Can you work these out from the model? Positions are in its coordinate system, mm. A direction names the side the tool comes from. Round coordinates to 2 decimals unless told otherwise and drop trailing zeros. Order: outer loops, then holes, each group sorted by start corner. A loop starts at its lowest first (then second) coordinate and runs counter-clockwise, first axis right, second up.
from build123d import *

# Parameters (mm, degrees)
SKETCH1_W           = 31.5
SKETCH1_H           = 30.3
SKETCH1_W_2         = 25.5
SKETCH1_H_2         = 24.3
BOSS_EXTRUDE1_DEPTH = 6
SKETCH2_W           = 31.5
SKETCH2_H           = 30.3
BOSS_EXTRUDE2_DEPTH = 2
CUT_EXTRUDE1_DEPTH  = 61
BOSS_EXTRUDE3_DEPTH = 2
SKETCH5_W           = 4
SKETCH5_H           = 27.3
BOSS_EXTRUDE4_DEPTH = 38
CUT_EXTRUDE2_DEPTH  = 38
SKETCH7_R           = 2.6
CUT_EXTRUDE3_DEPTH  = 38
CUT_EXTRUDE4_DEPTH  = 38
FILLET1_R           = 10


with BuildPart() as part:
    # Sketch1 → Boss-Extrude1 (new body)
    with BuildSketch(Plane.XY):
        with Locations((12.75, 12.15)):
            Rectangle(SKETCH1_W, SKETCH1_H)
        with Locations((12.75, 12.15)):
            Rectangle(SKETCH1_W_2, SKETCH1_H_2, mode=Mode.SUBTRACT)
    extrude(amount=BOSS_EXTRUDE1_DEPTH)

    # Sketch2 → Boss-Extrude2 (add)
    with BuildSketch(Plane(origin=(0, 0, 0), x_dir=(-1, 0, 0), z_dir=(0, 0, -1))):
        with Locations((-12.75, 12.15)):
            Rectangle(SKETCH2_W, SKETCH2_H)
    extrude(amount=BOSS_EXTRUDE2_DEPTH)

    # Sketch3 → Cut-Extrude1 (cut)
    with BuildSketch(Plane.XY.offset(6)):
        Polygon((-3, 24.391972576), (-3, 27.3), (28.5, 27.3), (28.5, 24.391972576), (28.5, 24.3), (0, 24.3), (-3, 24.3), align=None)
    extrude(amount=-CUT_EXTRUDE1_DEPTH, mode=Mode.SUBTRACT)

    # Sketch4 → Boss-Extrude3 (add)
    with BuildSketch(Plane.XY.offset(6)):
        with BuildLine():
            Line((-3, 24.3), (5.5, 24.3))
            Line((5.5, 24.3), (5.5, 8.75))
            ThreePointArc((5.5, 8.75), (12.75, 1.5), (20, 8.75))
            Line((20, 8.75), (20, 24.3))
            Line((20, 24.3), (28.5, 24.3))
            Line((28.5, 24.3), (28.5, -3))
            Line((28.5, -3), (-3, -3))
            Line((-3, -3), (-3, 24.3))
        make_face()
    extrude(amount=BOSS_EXTRUDE3_DEPTH)

    # Sketch5 → Boss-Extrude4 (add)
    with BuildSketch(Plane(origin=(0, 0, -2), x_dir=(-1, 0, 0), z_dir=(0, 0, -1))):
        with Locations((-26.5, 10.65)):
            Rectangle(SKETCH5_W, SKETCH5_H)
    extrude(amount=BOSS_EXTRUDE4_DEPTH)

    # Sketch6 → Cut-Extrude2 (cut)
    with BuildSketch(Plane.ZY.offset(-24.5)):
        with BuildLine():
            Line((-2, -3), (-40, -3))
            Line((-40, -3), (-40, 24.3))
            Line((-40, 24.3), (-2, 24.3))
            Line((-2, 24.3), (-17.826401454, 15.23386068))
            ThreePointArc((-17.826401454, 15.23386068), (-18.562622883, 14.501365189), (-18.832265792, 13.498437306))
            Line((-18.832265792, 13.498437306), (-18.832265792, 7.801562694))
            ThreePointArc((-18.832265792, 7.801562694), (-18.562622883, 6.798634811), (-17.826401454, 6.06613932))
            Line((-17.826401454, 6.06613932), (-2, -3))
        make_face()
    extrude(amount=-CUT_EXTRUDE2_DEPTH, mode=Mode.SUBTRACT)

    # Sketch7 → Cut-Extrude3 (cut)
    with BuildSketch(Plane.ZY.offset(-24.5)):
        with Locations(Location((-10.416132896, 10.65, 0), (0, 0, 270))):
            Circle(SKETCH7_R)
    extrude(amount=-CUT_EXTRUDE3_DEPTH, mode=Mode.SUBTRACT)

    # Sketch8 → Cut-Extrude4 (cut)
    with BuildSketch(Plane.ZY.offset(-24.5)):
        with BuildLine():
            ThreePointArc((-11.252656387, 0.614520451), (-15.36913817, 13.404749459), (-6.531723112, 23.52579068))
            Line((-6.531723112, 23.52579068), (-21.13731595, 18.385251799))
            Line((-21.13731595, 18.385251799), (-20.671768388, 0.766067146))
            Line((-20.671768388, 0.766067146), (-11.252656387, 0.614520451))
        make_face()
    extrude(amount=-CUT_EXTRUDE4_DEPTH, mode=Mode.SUBTRACT)

    # Fillet1
    fillet1_edges = [part.edges().sort_by_distance(p)[0] for p in [
        (26.5, 3.7451865, -13.774805753),
        (26.5, 17.5548135, -13.774805753),
    ]]
    fillet(fillet1_edges, radius=FILLET1_R)


solid = part.part
(1) I want a section at B-B, the plane x = 18. List the corners of the cut face in (y, z) for me, plus the area to 3 significant figures.
(2) I want a section at D-D, the plane z = -7. List the corners of the cut face in (x, y) for me, plus the area to 3 significant figures.
(3) I'm going to push flat-ended pins straight in: pin 1 Ø1.5 at (y, z) = (18.5, -11.5) entering from -X; pin 2 Ø7.5 at (x, y) = (12.5, 17) entering from -Z; pin 3 Ø5 at (x, z) = (14.5, -6.5) entering from -Y. Where does each tip first touch, or does it pass through?
(4) I want a section at C-C, the plane y = 16.5. List the corners of the cut face in (x, z) for me.
(5) I want a section at A-A, the plane z = 0.75. List the corners of the cut face in (x, y) for me, plus the area to 3 significant figures.
(6) On a 3-axis mill with a long thin cutter (end or side, diameter ignored), from which of +Z, -Z, +X, -X, +Y, -Y can I reach the whole of each face in a straight line? I mean faces 1 (the face through (5.5, 17, 7)), 2 (the face through (11, 11, -2)), 3 (the face through (21, 12, 6)). Say none if no direction works.
(7) Please list where these lines run through material, in increasing order: probe 1 along Z at (x, y) = (20.5, 19.75); probe 2 along Z at (x, y) = (26.8, 10.65); probe 3 along X at (y, z) = (0, -5.5).
(8) If we mould it in two halves opening along X, with no side actions, what happens to faces 4 (the face through (28.5, 10, -1)), 5 (the face through (13, 0, 3)), 6 (the face through (-3, 10, 3)), 7 (the face through (13, -3, 3))? For each: pulls with the +X half, pulls with the -X half, needs draft (parallel to the pull), parting line crosses it, or undercut.
Ans:
1. outline: (-3, -2) - (24.3, -2) - (24.3, 0) - (0, 0) - (0, 6) - (3.75, 6) - (3.75, 8) - (-3, 8) - close
1. area: 86.1 mm2
2. outline: (24.5, -0.14) - (28.5, -0.14) - (28.5, 21.44) - (24.5, 21.44) - close
2. area: 86.3 mm2
3. pin 1: stops at x = 24.5
3. pin 2: stops at z = -2
3. pin 3: passes through
4. outline: (-3, -2) - (24.5, -2) - (24.5, -13.79) - (28.5, -13.79) - (28.5, 8) - (20, 8) - (20, 6) - (25.5, 6) - (25.5, 0) - (0, 0) - (0, 6) - (5.5, 6) - (5.5, 8) - (-3, 8) - close
5. outline: (-3, -3) - (28.5, -3) - (28.5, 24.3) - (25.5, 24.3) - (25.5, 0) - (0, 0) - (0, 24.3) - (-3, 24.3) - close
5. area: 240 mm2
6. face 1: +Z, +Y
6. face 2: -Z, -X, +Y, -Y
6. face 3: +Y
7. probe 1: z = -2 to 0, 6 to 8
7. probe 2: z = -15.65 to -13.02, -7.82 to 8
7. probe 3: x = 24.5 to 28.5
8. face 4: pulls with the +X half
8. face 5: undercut
8. face 6: pulls with the -X half
8. face 7: needs draft
